Check sheet for the modelled part. Datum: model origin and axes. Units: mm. A direction names the side the tool comes from. Give positions to 0.01 mm unless a question says otherwise; leave off trailing zeros. Loops run counter-clockwise (first coordinate to the right, second up) from the corner with the lowest first, then second, coordinate; pieces in that order, holes last. Notation, with made-up numbers: (27.25, -9.5) - (58.25, -9.5) arc R5 cw to (58.25, -0.5) - close; hole circle Ø5 at (-18, 60.25). An arc over 180 degrees is marked (long way). Use one line per item in the form item = value.
from build123d import *

# Parameters (mm, degrees)
SKETCH1_W           = 25
SKETCH1_H           = 45
BOSS_EXTRUDE1_DEPTH = 30
SKETCH2_W           = 20.5
SKETCH2_H           = 40.5
CUT_EXTRUDE1_DEPTH  = 28
SKETCH3_W           = 20
SKETCH3_H           = 7.75
BOSS_EXTRUDE2_DEPTH = 3
SKETCH5_W           = 8
SKETCH5_H           = 28
CUT_EXTRUDE2_DEPTH  = 2.25
FILLET1_R           = 2
SKETCH6_R           = 2.15
CUT_EXTRUDE3_DEPTH  = 4
FILLET2_R           = 5
SKETCH8_W           = 30
SKETCH8_H           = 45
BOSS_EXTRUDE3_DEPTH = 10.5
SKETCH13_W          = 6
SKETCH13_H          = 45
BOSS_EXTRUDE6_DEPTH = 8
FILLET4_START       = -20.219298246
FILLET4_DEPTH       = 45
FILLET4_START_2     = -27.458286573
FILLET4_2_DEPTH     = 9.488988327
FILLET4_START_3     = 22.530701754
FILLET4_3_DEPTH     = 9.488988328
FILLET4_START_4     = -1
FILLET4_4_OUTLINE_W = 0.25
FILLET4_4_OUTLINE_H = 40.5
FILLET4_4_DEPTH     = 1
SKETCH14_R          = 3.25
BOSS_EXTRUDE7_DEPTH = 6


with BuildPart() as part:
    # Sketch1 → Boss-Extrude1 (new body)
    with BuildSketch(Plane.XY):
        with Locations((-0.657894737, 2.280701754)):
            Rectangle(SKETCH1_W, SKETCH1_H)
    extrude(amount=BOSS_EXTRUDE1_DEPTH)

    # Sketch2 → Cut-Extrude1 (cut)
    with BuildSketch(Plane(origin=(0, 0, 0), x_dir=(-1, 0, 0), z_dir=(0, 0, -1))):
        with Locations((0.657894737, 2.280701754)):
            Rectangle(SKETCH2_W, SKETCH2_H)
    extrude(amount=-CUT_EXTRUDE1_DEPTH, mode=Mode.SUBTRACT)

    # Sketch3 → Boss-Extrude2 (add)
    with BuildSketch(Plane(origin=(0, 0, 0), x_dir=(-1, 0, 0), z_dir=(0, 0, -1))):
        with Locations((0.657894737, 28.655701754)):
            Rectangle(SKETCH3_W, SKETCH3_H)
        with Locations((0.657894737, -24.094298246)):
            Rectangle(SKETCH3_W, SKETCH3_H)
    extrude(amount=-BOSS_EXTRUDE2_DEPTH)

    # Sketch5 → Cut-Extrude2 (cut)
    with BuildSketch(Plane(origin=(0, -17.969298246, 0), x_dir=(1, 0, 0), z_dir=(0, 1, 0))):
        with Locations((-0.657894737, -14)):
            Rectangle(SKETCH5_W, SKETCH5_H)
    extrude(amount=-CUT_EXTRUDE2_DEPTH, mode=Mode.SUBTRACT)

    # Fillet1
    fillet1_edges = [part.edges().sort_by_distance(p)[0] for p in [
        (-4.657894737, -20.219298246, 1.5),
        (3.342105263, -20.219298246, 1.5),
    ]]
    fillet(fillet1_edges, radius=FILLET1_R)

    # Sketch6 → Cut-Extrude3 (cut)
    with BuildSketch(Plane(origin=(0, 0, 0), x_dir=(-1, 0, 0), z_dir=(0, 0, -1))):
        with Locations((-4.092105263, 27.030701754)):
            Circle(SKETCH6_R)
        with Locations((5.407894737, 27.030701754)):
            Circle(SKETCH6_R)
        with Locations((5.407894737, -22.469298246)):
            Circle(SKETCH6_R)
        with Locations((-4.092105263, -22.469298246)):
            Circle(SKETCH6_R)
    extrude(amount=-CUT_EXTRUDE3_DEPTH, mode=Mode.SUBTRACT)

    # Fillet2
    fillet2_edges = [part.edges().sort_by_distance(p)[0] for p in [
        (9.342105263, 32.530701754, 1.5),
        (-10.657894737, 32.530701754, 1.5),
        (9.342105263, -27.969298246, 1.5),
        (-10.657894737, -27.969298246, 1.5),
    ]]
    fillet(fillet2_edges, radius=FILLET2_R)

    # Sketch8 → Boss-Extrude3 (add)
    with BuildSketch(Plane(origin=(11.842105263, 0, 0), x_dir=(0, 0, -1), z_dir=(1, 0, 0))):
        with Locations((-15, 2.280701754)):
            Rectangle(SKETCH8_W, SKETCH8_H)
    extrude(amount=BOSS_EXTRUDE3_DEPTH)

    # Sketch13 → Boss-Extrude6 (add)
    with BuildSketch(Plane(origin=(0, 0, 0), x_dir=(-1, 0, 0), z_dir=(0, 0, -1))):
        with Locations((-19.342105263, 2.280701754)):
            Rectangle(SKETCH13_W, SKETCH13_H)
    extrude(amount=BOSS_EXTRUDE6_DEPTH)

    # Fillet4: read off the stored shape, not the designer's step
    # Fillet4 outline → Fillet4 (add)
    with BuildSketch(Plane(origin=(0, 0, 0), x_dir=(1, 0, 0), z_dir=(0, 1, 0)).offset(FILLET4_START)):
        with BuildLine():
            Line((9.342105263, 0.399404936), (9.342105263, 0))
            Line((9.342105263, 0), (16.342105263, 0))
            Line((16.342105263, 0), (16.342105263, 8))
            ThreePointArc((16.342105263, 8), (13.899861657, 3.225529433), (9.342105263, 0.399404936))
        make_face()
    extrude(amount=FILLET4_DEPTH)

    # Fillet4 2 outline → Fillet4 2 (add)
    with BuildSketch(Plane(origin=(0, 0, 0), x_dir=(1, 0, 0), z_dir=(0, 1, 0)).offset(FILLET4_START_2)):
        with BuildLine():
            Line((6.544146292, 0), (9.342105263, 0))
            Line((9.342105263, 0), (9.342105263, 0.399404936))
            ThreePointArc((9.342105263, 0.399404936), (7.957307527, 0.100354788), (6.544146292, 0))
        make_face()
    extrude(amount=FILLET4_2_DEPTH)

    # Fillet4 3 outline → Fillet4 3 (add)
    with BuildSketch(Plane(origin=(0, 0, 0), x_dir=(1, 0, 0), z_dir=(0, 1, 0)).offset(FILLET4_START_3)):
        with BuildLine():
            Line((6.544146292, 0), (9.342105263, 0))
            Line((9.342105263, 0), (9.342105263, 0.399404936))
            ThreePointArc((9.342105263, 0.399404936), (7.957307527, 0.100354788), (6.544146292, 0))
        make_face()
    extrude(amount=FILLET4_3_DEPTH)

    # Fillet4 4 outline → Fillet4 4 (cut)
    with BuildSketch(Plane.XY.offset(FILLET4_START_4)):
        with BuildLine():
            Line((9.342105263, -27.458286573), (9.342105263, -22.969298246))
            ThreePointArc((9.342105263, -22.969298246), (8.58534724, -25.614085104), (6.544146253, -27.458286493))
            Line((6.544146253, -27.458286493), (9.342105263, -27.458286573))
        make_face()
        with BuildLine():
            Line((9.342105263, 32.019690082), (6.544146252, 32.019690001))
            ThreePointArc((6.544146252, 32.019690001), (8.58534724, 30.175488613), (9.342105263, 27.530701754))
            Line((9.342105263, 27.530701754), (9.342105263, 32.019690082))
        make_face()
        with Locations((9.467105263, 2.280701754)):
            Rectangle(FILLET4_4_OUTLINE_W, FILLET4_4_OUTLINE_H)
    extrude(amount=FILLET4_4_DEPTH, mode=Mode.SUBTRACT)

    # Sketch14 → Boss-Extrude7 (add)
    with BuildSketch(Plane(origin=(22.342105263, 0, 0), x_dir=(0, 0, -1), z_dir=(1, 0, 0))):
        with Locations(Location((-21.156070928, 14.873665711, 0), (0, 0, 90))):
            Circle(SKETCH14_R)
        with Locations(Location((3.643929072, 15.073774065, 0), (0, 0, 90))):
            Circle(SKETCH14_R)
        with Locations(Location((3.643929072, -9.726225935, 0), (0, 0, 90))):
            Circle(SKETCH14_R)
        with Locations(Location((-21.156070928, -9.726225935, 0), (0, 0, 90))):
            Circle(SKETCH14_R)
    extrude(amount=BOSS_EXTRUDE7_DEPTH)


solid = part.part
Item 1: Thickness scan on L1, parallel to Y at x = 5.5, z = 13.5; L2, parallel to X at y = 1, z = 16; L3, parallel to Z at x = 1, y = 23.5. Record the ranges inside material, lowest first.
Answer block:
L1 = -20.22 to -17.97, 22.53 to 24.78
L2 = -13.16 to -10.91, 9.59 to 22.34
L3 = 0 to 30
Item 2: Gauge pin test, flat ends, axial feed: P1, Ø10, axis at x = 22, z = 18, coming from the +Y side; P2, Ø5, axis at x = 4.09, y = 27.03, coming from the -Z side; P3, Ø6, axis at x = 2, z = 11.5, coming from the -Y side. Record the tip position at first contact, or that the pin passes through.
Answer block:
P1 = 24.78
P2 = 0
P3 = -20.22
Item 3: Section check B-B on y = -14. Record the boundary of the cut face in (x, z).
Answer block:
outline = (-13.16, 0) - (-10.91, 0) - (-10.91, 28) - (9.59, 28) - (9.59, -0.48) arc R10 cw to (16.34, -8) - (22.34, -8) - (22.34, 30) - (-13.16, 30) - close
Item 4: Section check A-A on x = 0. Record the boundary of the cut face in (y, z).
Answer block:
outline = (-27.97, 0) - (-20.22, 0) - (-20.22, 3) - (-27.97, 3) - close; (-20.22, 28) - (22.53, 28) - (22.53, 0) - (32.53, 0) - (32.53, 3) - (24.78, 3) - (24.78, 30) - (-20.22, 30) - close
Item 5: Mould release check, pull along Z, two halves, no side actions. Record for faces 1 (the face through (3.342, -19, 14)), 2 (the face through (4, 24.781, 15)), 3 (the face through (4, 2, 30)): released by +Z, released by -Z, zero draft, split by the parting line, or undercut.
Answer block:
face_1 = undercut
face_2 = zero draft
face_3 = released by +Z
Item 6: Section check C-C on z = 12.5. Record the boundary of the cut face in (x, y), then the cut area to 3 significant figures.
Answer block:
outline = (-13.16, -20.22) - (-4.66, -20.22) - (-4.66, -17.97) - (-10.91, -17.97) - (-10.91, 22.53) - (9.59, 22.53) - (9.59, -17.97) - (3.34, -17.97) - (3.34, -20.22) - (22.34, -20.22) - (22.34, 24.78) - (-13.16, 24.78) - close
area = 749 mm2
Item 7: Access from +Z, -Z, +X, -X, +Y, -Y to the whole of each face (thin tool, end or side, straight path). Record for faces 4 (the face through (9.592, 2, 14)), 5 (the face through (-10.658, 26, 1)), 6 (the face through (-11.4, -0.1, 0)), 7 (the face through (22.342, 2, 11)).
Answer block:
face_4 = -Z
face_5 = +Z, -Z, -X, +Y
face_6 = -Z, -X, +Y, -Y
face_7 = +X
Item 8: Section check D-D on x = 26. Record the boundary of the cut face in (y, z), then the cut area to 3 significant figures.
Answer block:
outline = circle Ø6.5 at (-9.73, -3.64); circle Ø6.5 at (-9.73, 21.16); circle Ø6.5 at (14.87, 21.16); circle Ø6.5 at (15.07, -3.64)
area = 133 mm2
